from build123d import *

# Parameters (mm, degrees)
CUT_EXTRUDE1_DEPTH = 10


with BuildPart() as part:
    # Sketch1 → Revolve1 (revolve)
    with BuildSketch(Plane.XY):
        Polygon((60.5, 0), (15, 0), (15, 4), (58.5, 4), (58.5, 10), (60, 10), (60, 140), (62.5, 140), (62.5, 8), (60.5, 8), align=None)
    revolve(axis=Axis((0, 0, 0), (0, 1, 0)))

    # Sketch2 → Cut-Extrude1 (cut)
    with BuildSketch(Plane(origin=(0, 4, 0), x_dir=(1, 0, 0), z_dir=(0, 1, 0))):
        with BuildLine():
            ThreePointArc((19.595917942, -4), (14.142135624, -14.142135624), (4, -19.595917942))
            Line((4, -19.595917942), (4, -58.36308765))
            ThreePointArc((4, -58.36308765), (41.365746699, -41.365746699), (58.36308765, -4))
            Line((58.36308765, -4), (19.595917942, -4))
        make_face()
        with BuildLine():
            Line((22.386980793, 54.046952652), (7.653668647, 18.47759065))
            ThreePointArc((7.653668647, 18.47759065), (15.428387799, 12.726541161), (19.595917942, 4))
            Line((19.595917942, 4), (58.36308765, 4))
            ThreePointArc((58.36308765, 4), (47.500713214, 34.145750016), (22.386980793, 54.046952652))
        make_face()
        with BuildLine():
            ThreePointArc((-19.595917942, 4), (-15.428387799, 12.726541161), (-7.653668647, 18.47759065))
            Line((-7.653668647, 18.47759065), (-22.386980793, 54.046952652))
            ThreePointArc((-22.386980793, 54.046952652), (-47.500713214, 34.145750016), (-58.36308765, 4))
            Line((-58.36308765, 4), (-19.595917942, 4))
        make_face()
        with BuildLine():
            Line((-4, -58.36308765), (-4, -19.595917942))
            ThreePointArc((-4, -19.595917942), (-14.142135624, -14.142135624), (-19.595917942, -4))
            Line((-19.595917942, -4), (-58.36308765, -4))
            ThreePointArc((-58.36308765, -4), (-41.365746699, -41.365746699), (-4, -58.36308765))
        make_face()
    extrude(amount=-CUT_EXTRUDE1_DEPTH, mode=Mode.SUBTRACT)


solid = part.part
Input: part model. Units: mm. Frame: model coordinates. A direction names the side the tool comes from. Coordinates: 2 decimals unless noted, no trailing zeros. Write each loop counter-clockwise with the first axis right and the second up, starting at its lowest first coordinate (ties: lowest second). Pieces come first, ordered by that corner, then holes. Notation, with made-up numbers: M -3,-16.5 L 24,-16.5 A17 cw 24,16.5 Z; hole C 10,60 d2. An arc over 180 degrees is marked long. Answer as a JSON object with one key per item and string values. Group by question number.
(1) Section C-C on x = 0. Output: boundary loops of the cut face in (y, z), plus the area to 3 significant figures.
(2) Contact query for flat-ended pins moving along their axis: P1, Ø10, axis at x = -2.5, y = 61, coming from the -Z side; P2, Ø4.5, axis at y = 3, z = 32.5, coming from the +X side; P3, Ø1.5, axis at x = 13, z = -5, coming from the -Y side; P4, Ø2, axis at x = -33, y = 2, coming from the +Z side. Output: stop coordinate, or through.
(3) Section A-A on z = 0. Output: boundary loops of the cut face in (x, y).
(4) Ray query, line 1 along X through (y, z) = (3.1, 0); line 2 along Z through (x, y) = (0, 102). Return the intervals inside material, ascending. Write a range as [from, to].
(5) Mould query, pull axis Z, two halves, no side actions, for faces 5 (the face through (0, 0, -18)), 6 (the face through (-62.44, 73.08, -2.75)), 7 (the face through (-14.985, 2.028, -0.66)). Classes: pulls with the +Z half, pulls with the -Z half, needs draft (parallel to the pull), parting line crosses it, or undercut.
(6) Set-up query: faces 1 (the face through (-59.94, 75.91, -2.64)), 2 (the face through (15.123, 2.028, -36.511)), 3 (the face through (56, 140, -23)), 4 (the face through (-13.12, 3.94, 59.06)). Return all of +Z, -Z, +X, -X, +Y, -Y with unobstructed straight access to the full face (end or side cutting, diameter ignored); none if empty.
(7) Section D-D on z = -31.5. Output: boundary loops of the cut face in (x, y), plus the area to 3 significant figures.
(8) Section B-B on x = -32. Output: boundary loops of the cut face in (y, z).
Result set:
{
 "1": {"outline": "M 0,-60.5 L 8,-60.5 L 8,-62.5 L 140,-62.5 L 140,-60 L 10,-60 L 10,-58.5 L 4,-58.5 L 4,-15 L 0,-15 Z; M 0,15 L 4,15 L 4,58.5 L 10,58.5 L 10,60 L 140,60 L 140,62.5 L 8,62.5 L 8,60.5 L 0,60.5 Z", "area": "1,050 mm2"},
 "2": {"P1": "stops at z = -62.5", "P2": "stops at x = 52.39", "P3": "passes through", "P4": "stops at z = 51.34"},
 "3": {"outline": "M -62.5,8 L -60.5,8 L -60.5,0 L -15,0 L -15,4 L -58.5,4 L -58.5,10 L -60,10 L -60,140 L -62.5,140 Z; M 15,0 L 60.5,0 L 60.5,8 L 62.5,8 L 62.5,140 L 60,140 L 60,10 L 58.5,10 L 58.5,4 L 15,4 Z"},
 "4": {"line 1": "x = [-60.5, -15], [15, 60.5]", "line 2": "z = [-62.5, -60], [60, 62.5]"},
 "5": {"face 5": "needs draft", "face 6": "parting line crosses it", "face 7": "undercut"},
 "6": {"face 1": "+Y", "face 2": "+Y, -Y", "face 3": "+Z, -Z, +X, -X, +Y", "face 4": "-Y"},
 "7": {"outline": "M -53.98,8 L -51.65,8 L -51.65,0 L -49.3,0 L -49.3,10 L -51.07,10 L -51.07,140 L -53.98,140 Z; M -13.05,0 L 13.05,0 L 13.05,4 L -13.05,4 Z; M 49.3,0 L 51.65,0 L 51.65,8 L 53.98,8 L 53.98,140 L 51.07,140 L 51.07,10 L 49.3,10 Z", "area": "919 mm2"},
 "8": {"outline": "M 0,-51.34 L 8,-51.34 L 8,-53.69 L 140,-53.69 L 140,-50.75 L 10,-50.75 L 10,-48.97 L 0,-48.97 Z; M 0,-4 L 4,-4 L 4,4 L 0,4 Z; M 0,48.97 L 10,48.97 L 10,50.75 L 140,50.75 L 140,53.69 L 8,53.69 L 8,51.34 L 0,51.34 Z"}
}
